Autodesk Inventor part; units mm, degrees
ref_plane "YZ Plane" through (0, 0, 0) normal (1, 0, 0) x (0, 1, 0)
ref_plane "XZ Plane" through (0, 0, 0) normal (0, 1, 0) x (-1, 0, 0)
ref_plane "XY Plane" through (0, 0, 0) normal (0, 0, 1) x (1, 0, 0)
sketch "Sketch1" plane through (0, 0, 0) normal (0, 1, 0) x (-1, 0, 0)
  circle A0 centre (0, 0) radius 60
  circle A1 centre (60, 0) radius 7.5
  circle A2 centre (-30, 51.9615) radius 7.5
  circle A3 centre (-30, -51.9615) radius 7.5
  circle A4 centre (0, -35) radius 12
  line L0 (0, -118.7756) -> (0, 118.7756)
  line L1 (121.2, 0) -> (-90.2, 0)
  circle A5 centre (0, 35) radius 12
  line L2 (21, 10) -> (-21, 10)
  line L3 (-21, 10) -> (-21, 60)
  line L4 (-21, 60) -> (21, 60)
  line L5 (21, 60) -> (21, 10)
  line L6 (21, 10) -> (-21, 60) construction
  line L7 (-21, 10) -> (21, 60) construction
  line L8 (21, -60) -> (-21, -60)
  line L9 (-21, -60) -> (-21, -10)
  line L10 (-21, -10) -> (21, -10)
  line L11 (21, -10) -> (21, -60)
  line L12 (21, -60) -> (-21, -10) construction
  line L13 (-21, -60) -> (21, -10) construction
  circle A6 centre (60, 0) radius 15
  circle A7 centre (-30, 51.9615) radius 15
  circle A8 centre (-30, -51.9615) radius 15
  circle A9 centre (56, 49.8397) radius 35
  circle A10 centre (56, -49.8397) radius 35
  circle A11 centre (0, 0) radius 5.15
  circle A12 centre (16, 55) radius 5
  circle A13 centre (16, -55) radius 5
  circle A14 centre (-14.8343, -65) radius 5
  circle A15 centre (-14.8343, 65) radius 5
  line L14 (-30, -36.9615) -> (-30, 36.9615)
  circle A16 centre (-35, -32.5966) radius 5
  circle A17 centre (-35, 32.5966) radius 5
  circle A18 centre (0, -8) radius 1.75
  circle A19 centre (8, 0) radius 1.75
  circle A20 centre (0, 8) radius 1.75
  circle A21 centre (-8, 0) radius 1.75
  line L15 (0, -9.75) -> (0, -10)
  point P0 (58.8, 14.9519)
  point P1 (21, 49.8397)
  point P2 (21, 55)
  point P3 (16, 60)
  point P4 (-16.174, 57.7789)
  point P5 (-21, 56.3204)
  point P6 (-21, -56.3204)
  point P7 (16, -60)
  point P8 (21, -55)
  point P9 (21, -49.8397)
  point P10 (58.8, -14.9519)
  point P11 (20.8372, -56.2655)
  point P12 (21, -56.205)
  point P13 (12.5965, -58.6628)
  point P14 (0, -60)
  point P15 (20.8372, 56.2655)
  point P16 (21, 56.205)
  point P17 (12.5965, 58.6628)
  point P18 (-21, -39.9615)
  point P19 (0, -10)
  point P20 (0, -5.15)
  point P21 (-5.15, 0)
  point P22 (-21, -56.205)
  point P23 (-16.174, -57.7789)
  point P24 (0, -60)
  point P25 (0, -47)
  point P26 (0, -23)
  point P27 (0, 5.15)
  point P28 (0, 10)
  point P29 (-21, 39.9615)
  point P30 (0, 60)
  point P31 (0, 23)
  point P32 (0, 47)
  point P33 (0, 60)
  point P34 (5.15, 0)
  point P35 (45, 0)
  point P36 (21.546, -55.9979)
  point P37 (58.1195, -14.904)
  point P38 (58.125, -14.8824)
  point P39 (58.1195, 14.904)
  point P40 (21.546, 55.9979)
  point P41 (58.125, 14.8824)
  point P42 (-60, 0)
  point P43 (-41.951, -42.8966)
  point P44 (-23.2831, -55.2982)
  point P45 (-36.2481, -47.8129)
  point P46 (-36.2481, 47.8129)
  point P47 (-23.2831, 55.2982)
  point P48 (-21, 56.205)
  point P49 (75, 0)
  point P50 (59.5312, 7.4853)
  point P51 (67.5, 0)
  point P52 (59.5312, -7.4853)
  point P53 (52.5, 0)
  point P54 (60, 0)
  point P55 (-41.951, 42.8966)
  point P56 (-17.3358, -60)
  point P57 (-17.3358, 60)
  point P58 (-14.8343, 60)
  point P59 (-18.6257, 61.7404)
  point P60 (-33.75, 37.4378)
  point P61 (-30, 32.5966)
  point P62 (-30, -32.5966)
  point P63 (-33.75, -37.4378)
  point P64 (-18.6257, -61.7404)
  point P65 (-14.8343, -60)
  point P66 (-30, 0)
  dimension "d0" = 120
  dimension "d13" = 30
  dimension "d14" = 30
  dimension "d28" = 3.5
  dimension "d1" = 15
  dimension "d4" = 360
  dimension "d6" = 24
  dimension "d7" = 35
  dimension "d8" = 42
  dimension "d9" = 50
  dimension "d10" = 42
  dimension "d11" = 50
  dimension "d12" = 30
  dimension "d15" = 70
  dimension "d16" = 10.3
  dimension "d19" = 10
  dimension "d20" = 10
  dimension "d23" = 10
  dimension "d24" = 10
  dimension "d25" = 30
  dimension "d26" = 10
  dimension "d27" = 10
  dimension "d29" = 8
  dimension "d32" = 360
extrude "Extrusion1" add sketch "Sketch1" along normal blind 3.5 contours A1 L1 A6 A0 | A0 A6 L1 A1 | A1 L1 A6 A0 | A0 A6 L1 A1 | A6 L1 A19 A11 L0 A20 L2 L5 A9 A0 | A0 A9 A6 | A6 A10 A0 | A0 A10 L11 L10 L0 A18 A11 L1 A19 A6 | L5 L2 L0 A5 A0 A12 | L11 A13 A0 L0 A4 L10 | A12 A0 | A13 A0 | A0 A12 | A0 L4 A12 | L2 L3 A7 A0 L0 A5 | L0 A20 A11 L1 A21 L14 A7 L3 L2 | A13 A0 | L10 L9 A8 L14 L1 A21 A11 L0 A18 | L0 A4 A0 A8 L9 L10 | A13 L8 A0 | A0 A7 L4 | L8 A8 A0 | A7 L3 A0 | A0 L3 L4 A7 | L4 A7 A15 | A7 A0 A2 L3 | A8 A0 L9 | L9 A0 A3 A8 | A8 L8 L9 A0 | A14 A8 L8 | A0 A2 A7 L4 L3 | L14 A17 A7 | L9 L8 A8 A0 A3 | A8 A16 L14
sketch "Sketch2" plane through (0, 3.5, 0) normal (0, 1, 0) x (1, 0, 0)
  circle A0 centre (0, -35) radius 12
  line L0 (-99, 0) -> (69, 0)
  point P0 (0, 0)
  point P1 (15.5, -50.5)
  point P2 (-15.5, -50.5)
  point P3 (-15.5, -19.5)
  point P4 (15.5, -19.5)
  point P5 (15.5, 50.5)
  point P6 (-15.5, 50.5)
  point P7 (-15.5, 19.5)
  point P8 (15.5, 19.5)
  dimension "d34" = 15.5
  dimension "d35" = 31
  dimension "d36" = 15.5
  dimension "d37" = 31
hole "Hole1" at (15.5, 3.5, 50.5) at (-15.5, 3.5, 50.5) at (-15.5, 3.5, 19.5) at (15.5, 3.5, 19.5) at (15.5, 3.5, -50.5) at (-15.5, 3.5, -50.5) at (-15.5, 3.5, -19.5) at (15.5, 3.5, -19.5) direction (0, -1, 0) diameter 3.05 end through all
properties part number "De_Tren" material "Aluminum 6061"
CAD build for the part. Positions are in the model's coordinates, mm. A direction names the side the tool comes from. Round coordinates to 2 decimals unless told otherwise and drop trailing zeros. Order: outer loops, then holes, each group sorted by start corner. A loop starts at its lowest first (then second) coordinate and runs counter-clockwise, first axis right, second up.
Q1. Slice it at A-A (z = 19.5). Write the cut outline in (x, y) (3 decimals).
Q2. Slice it at D-D (z = 0). Write the cut outline in (x, y).
Q3. Wall check: L1, parallel to Z at x = 0, y = 2.05; L2, parallel to X at y = 1, z = 19.5 (3 decimals); L3, parallel to Z at x = 15.5, y = 0.9 (3 decimals). Give the ranges that are in metal, low to high.
Q4. Which spindle directions (+Z, -Z, +X, -X, +Y, -Y) get a long thin tool onto all of the face, cutting with end or side? Do faces 1 (the flat face through (-21, 2, -52)), 2 (the cylindrical face through (-19, 2, 59)). Say none if no direction does.
Q5. Slice it at B-B (x = 0). Write the cut outline in (y, z).
Q6. Two-plate mould, pull along X, no slides. Class faces 3 (the cylindrical face through (42.52, 1.73, -60.22)), 4 (the cylindrical face through (-14.147, 1.726, -18.796)), 5 (the flat face through (-21, 2, 52)), 6 (the flat face through (-1, 3.5, -14)): pulls with the +X half, pulls with the -X half, needs draft (parallel to the pull), parting line crosses it, or undercut.
Q7. Slice it at C-C (y = 2.5). State how many separate pieces and enclosed holes the cut face has, and give its area (3 significant figures).
Q8. Drop flat-ended pins along their axis: pin 1 (1 mm diameter, centred on y = 1.5, z = -4, fed in from +X); pin 2 (1.5 mm diameter, centred on x = 31.5, y = 0.5, fed in from -Z); pin 3 (1 mm diameter, centred on x = -7.5, y = 2, fed in from +Z). Give the stop position or say it passes through.
Results below:
1. outline: (-38.55, 0) - (-17.025, 0) - (-17.025, 3.5) - (-38.55, 3.5) - close; (-13.975, 0) - (13.975, 0) - (13.975, 3.5) - (-13.975, 3.5) - close; (17.025, 0) - (30, 0) - (30, 3.5) - (17.025, 3.5) - close
2. outline: (-75, 0) - (-67.5, 0) - (-67.5, 3.5) - (-75, 3.5) - close; (-52.5, 0) - (-9.75, 0) - (-9.75, 3.5) - (-52.5, 3.5) - close; (-6.25, 0) - (-5.15, 0) - (-5.15, 3.5) - (-6.25, 3.5) - close; (5.15, 0) - (6.25, 0) - (6.25, 3.5) - (5.15, 3.5) - close; (9.75, 0) - (30, 0) - (30, 3.5) - (9.75, 3.5) - close
3. L1: z = -60 to -47, -23 to -9.75, -6.25 to -5.15, 5.15 to 6.25, 9.75 to 23, 47 to 60
3. L2: x = -38.55 to -17.025, -13.975 to 13.975, 17.025 to 30
3. L3: z = -60.045 to -52.025, -48.975 to -21.025, -17.975 to 17.975, 21.025 to 48.975, 52.025 to 60.045
4. face 1: -Z, -X, +Y, -Y
4. face 2: +Z, -X, +Y, -Y
5. outline: (0, -60) - (3.5, -60) - (3.5, -47) - (0, -47) - close; (0, -23) - (3.5, -23) - (3.5, -9.75) - (0, -9.75) - close; (0, -6.25) - (3.5, -6.25) - (3.5, -5.15) - (0, -5.15) - close; (0, 5.15) - (3.5, 5.15) - (3.5, 6.25) - (0, 6.25) - close; (0, 9.75) - (3.5, 9.75) - (3.5, 23) - (0, 23) - close; (0, 47) - (3.5, 47) - (3.5, 60) - (0, 60) - close
6. face 3: parting line crosses it
6. face 4: undercut
6. face 5: pulls with the -X half
6. face 6: needs draft
7. separate pieces: 1
7. enclosed holes: 18
7. area: 7,370 mm2
8. pin 1: stops at x = 30
8. pin 2: stops at z = -66.94
8. pin 3: stops at z = 60
